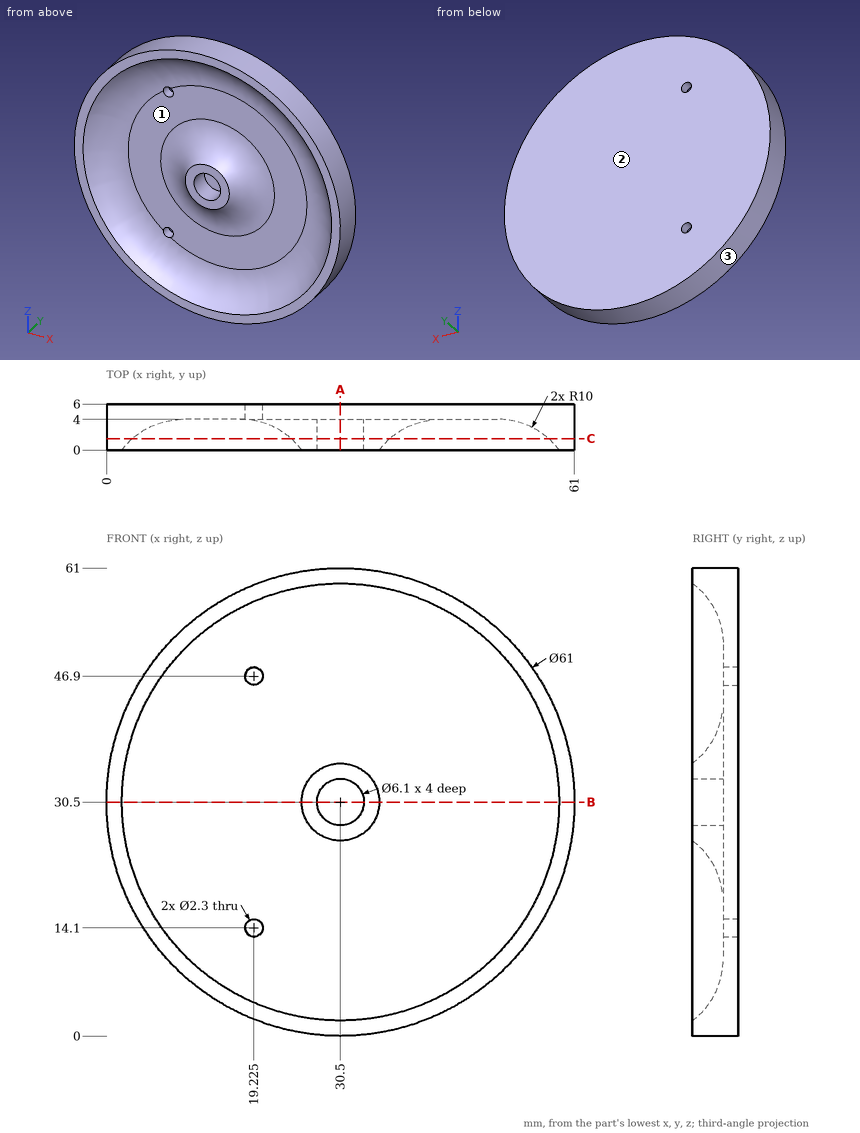
Job drawing, mm, ordinate dimensions from the low corner. One solid piece. Round coordinates to 2 decimals unless told otherwise and drop trailing zeros. Loops run counter-clockwise (first coordinate to the right, second up) from the corner with the lowest first, then second, coordinate; pieces in that order, holes last. Notation, with made-up numbers: M -25.75,-37.5 L 17.25,-37.5 A31 ccw 17.25,-12.5 Z; hole C -24.75,-9.5 d4. An arc over 180 degrees is marked long. Answer as CSV lines item,"result".
1. Cut at B-B on z = 30.5. Write the cut outline in (x, y).
Resolved:
outline,"M 0,0 L 2,0 A10 cw 10,4 L 17.45,4 A10 cw 25.45,0 L 27.45,0 L 27.45,4 L 33.55,4 L 33.55,0 L 35.55,0 A10 cw 43.55,4 L 51,4 A10 cw 59,0 L 61,0 L 61,6 L 0,6 Z"
2. Wall check: probe 1 along Y at (x, z) = (40, 13); probe 2 along X at (y, z) = (1, 44.5); probe 3 along X at (y, z) = (5.75, 46). Give the ranges that are in metal, low to high. Write a range as [from, to].
Resolved:
probe 1,"y = [4, 6]"
probe 2,"x = [3.4, 6.67], [54.33, 57.6]"
probe 3,"x = [4.23, 18.51], [19.94, 56.77]"
3. Cut at A-A on x = 30.5. Write the cut outline in (y, z), then the cut area to 3 significant figures.
Resolved:
outline,"M 0,0 L 6,0 L 6,61 L 0,61 L 0,59 A10 cw 4,51 L 4,43.55 A10 cw 0,35.55 L 0,33.55 L 4,33.55 L 4,27.45 L 0,27.45 L 0,25.45 A10 cw 4,17.45 L 4,10 A10 cw 0,2 Z"
area,"193 mm²"
4. Two-plate mould, pull along Z, no slides. Class the marked faces 1, 2 and 3: released by +Z, released by -Z, zero draft, split by the parting line, or undercut.
Resolved:
face 1,"undercut"
face 2,"zero draft"
face 3,"split by the parting line"
5. Cut at C-C on y = 1.5. Write the cut outline in (x, z).
Resolved:
outline,"C 30.5,30.5 d61; C 30.5,30.5 d12.87; hole C 30.5,30.5 d54.23; hole C 30.5,30.5 d6.1"
6. Flat gauge pins, fed straight in: P1, Ø5.5, axis at x = 30.5, z = 30.5, coming from the -Y side; P2, Ø12.5, axis at x = 36.5, z = 20.5, coming from the -Y side; P3, Ø3, axis at y = 3.5, z = 23.5, coming from the +X side. Where does each tip first touch, or does it go through?
Resolved:
P1,"stops at y = 4"
P2,"stops at y = 0.45"
P3,"stops at x = 60.5"
